```python
from build123d import *

# Parameters (mm, degrees)
BOSS_EXTRUDE1_DEPTH = 1.5875
BOSS_EXTRUDE2_REACH = 24.56
SKETCH3_W           = 1.5875
SKETCH3_H           = 7.003924561
SKETCH4_R           = 2
CUT_EXTRUDE1_DEPTH  = 15
SKETCH5_R           = 2
BOSS_EXTRUDE3_DEPTH = 1.5875


with BuildPart() as part:
    # Sketch2 → Boss-Extrude1 (new body)
    with BuildSketch(Plane.XY):
        Polygon((0, 0), (0, 94.86), (-6.6, 94.86), (-6.6, 5.71), (-22.56, 5.71), (-22.56, 94.86), (-29.16, 94.86), (-29.16, 0), align=None)
    extrude(amount=BOSS_EXTRUDE1_DEPTH)

    # Sketch3 → Boss-Extrude2 (add, up to next)
    with BuildSketch(Plane(origin=(-22.56, 0, 0), x_dir=(0, 0, -1), z_dir=(1, 0, 0)), mode=Mode.PRIVATE) as boss_extrude2_sk1:
        with Locations((-0.79375, 91.35803772)):
            Rectangle(SKETCH3_W, SKETCH3_H)
    boss_extrude2_tool1 = extrude(boss_extrude2_sk1.sketch, amount=BOSS_EXTRUDE2_REACH, mode=Mode.PRIVATE) - part.part
    add(boss_extrude2_tool1.solids().sort_by_distance((-22.56, 91.358038, 0.79375))[0])

    # Sketch4 → Cut-Extrude1 (cut)
    with BuildSketch(Plane.XY.offset(1.5875)):
        with Locations((-3.354353393, 47.428062363)):
            Circle(SKETCH4_R)
        with Locations((-25.771024386, 47.428062363)):
            Circle(SKETCH4_R)
        with Locations((-25.771024386, 3.86)):
            Circle(SKETCH4_R)
        with Locations((-3.354353393, 3.86)):
            Circle(SKETCH4_R)
        with Locations((-25.771024386, 74.86)):
            Circle(SKETCH4_R)
        with Locations((-3.354353393, 74.86)):
            Circle(SKETCH4_R)
    extrude(amount=-CUT_EXTRUDE1_DEPTH, mode=Mode.SUBTRACT)

    # Sketch5 → Boss-Extrude3 (add)
    with BuildSketch(Plane.XY.offset(1.5875)):
        with Locations((-25.771024386, 47.428062363)):
            Circle(SKETCH5_R)
        with Locations((-3.354353393, 47.428062363)):
            Circle(SKETCH5_R)
    extrude(amount=-BOSS_EXTRUDE3_DEPTH)


solid = part.part
```
Verification items for the finished model (mm, model axes). A direction names the side the tool comes from. Give positions to 0.01 mm unless a question says otherwise; leave off trailing zeros. Order: outer loops, then holes, each group sorted by start corner. A loop starts at its lowest first (then second) coordinate and runs counter-clockwise, first axis right, second up. Notation, with made-up numbers: M 55,30.5 L 97,30.5 A24 cw 97,57.5 Z; hole C 52,7 d11. An arc over 180 degrees is marked long. Return JSON: item names as keys, results as strings. Group by question number.
1) Scan lines: line 1 (X direction, y = 49, z = 0.5); line 2 (Y direction, x = -13, z = 0.95); line 3 (Y direction, x = -27, z = 1.25). Record each from-to range of solid material in increasing order.
2) Section check A-A on y = 74.86. Record the cut outline in (x, z), and give its area (4 significant figures).
3) Access from +Z, -Z, +X, -X, +Y, -Y to the whole of each face (thin tool, end or side, straight path). Record for faces 1 (the face through (-15, 0, 1)), 2 (the face through (-6.6, 47, 1)).
4) Section check D-D on y = 3.86. Record the cut outline in (x, z), and give its area (3 significant figures).
5) Section check B-B on x = -11. Record the cut outline in (y, z).
6) Mould release check, pull along X, two halves, no side actions. Record for faces 3 (the face through (-25, 47, 0)), 4 (the face through (0, 47, 1)), 5 (the face through (-29.16, 48, 1)), 6 (the face through (-14, 5.71, 1)): pulls with the +X half, pulls with the -X half, needs draft (parallel to the pull), parting line crosses it, or undercut.
7) Section check C-C on z = 1. Record the cut outline in (x, y), and give its area (3 significant figures).
8) Go/stop test with a flat-tipped pin: pin 1 Ø0.8 at (y, z) = (41.5, 1) entering from +X. Record where the tip stops, or that it passes through.
Answer block:
{
 "1": {"line 1": "x = -29.16 to -22.56, -6.6 to 0", "line 2": "y = 0 to 5.71, 87.86 to 94.86", "line 3": "y = 0 to 2.28, 5.44 to 73.28, 76.44 to 94.86"},
 "2": {"outline": "M -29.16,0 L -27.77,0 L -27.77,1.59 L -29.16,1.59 Z; M -23.77,0 L -22.56,0 L -22.56,1.59 L -23.77,1.59 Z; M -6.6,0 L -5.35,0 L -5.35,1.59 L -6.6,1.59 Z; M -1.35,0 L 0,0 L 0,1.59 L -1.35,1.59 Z", "area": "8.255 mm^2"},
 "3": {"face 1": "+Z, -Z, +X, -X, -Y", "face 2": "+Z, -Z"},
 "4": {"outline": "M -29.16,0 L -27.77,0 L -27.77,1.59 L -29.16,1.59 Z; M -23.77,0 L -5.35,0 L -5.35,1.59 L -23.77,1.59 Z; M -1.35,0 L 0,0 L 0,1.59 L -1.35,1.59 Z", "area": "33.6 mm^2"},
 "5": {"outline": "M 0,0 L 5.71,0 L 5.71,1.59 L 0,1.59 Z; M 87.86,0 L 94.86,0 L 94.86,1.59 L 87.86,1.59 Z"},
 "6": {"face 3": "needs draft", "face 4": "pulls with the +X half", "face 5": "pulls with the -X half", "face 6": "undercut"},
 "7": {"outline": "M -29.16,0 L 0,0 L 0,94.86 L -29.16,94.86 Z; hole C -25.77,3.86 d4; hole C -25.77,74.86 d4; hole M -22.56,5.71 L -6.6,5.71 L -6.6,87.86 L -22.56,87.86 Z; hole C -3.35,3.86 d4; hole C -3.35,74.86 d4", "area": "1,400 mm^2"},
 "8": {"pin 1": "stops at x = 0"}
}
